Part print with two shaded views. Sizes in mm from the minimum x, y, z corner. A direction names the side the tool comes from. Round coordinates to 2 decimals unless told otherwise and drop trailing zeros. Write each loop counter-clockwise with the first axis right and the second up, starting at its lowest first coordinate (ties: lowest second). Pieces come first, ordered by that corner, then holes. Notation, with made-up numbers: (-14, 53.5) - (0, 53.5) arc R17 ccw to (0, 71.5) - close; hole circle Ø6 at (73, 79.5). An arc over 180 degrees is marked (long way). Answer as a JSON object with one key per item and string values. Group by question number.
Item 1: Slice it at B-B, the plane x = 522.5. List the corners of the cut face in (y, z).
Item 2: Two-plate mould, pull along Y, no slides. Class the marked faces 3, 4, 5 and 6: +Y half, -Y half, draft (parallel to the pull), parting line (faces both ways), or undercut.
Item 3: Flat gauge pin, fed straight in: pin 1 (10 mm diameter, centred on x = 379.5, y = 118, fed in from +Z). Where does the tip first touch, or does it go through?
Item 4: Slice it at D-D, the plane x = 293.5. List the corners of the cut face in (y, z).
Item 5: Slice it at A-A, the plane y = 49. List the corners of the cut face in (x, z), then the cut area to 3 significant figures.
Item 6: Slice it at C-C, the plane z = 130.5. List the corners of the cut face in (x, y), then the cut area to 3 significant figures.
Item 7: Probe line 1 (Y direction, x = 104, z = 51); line 2 (X direction, y = 137.5, z = 66); line 3 (Z direction, x = 210.5, y = 37.5). List the from-to ranges inside material, lowest first. Write a range as from..to.
Item 8: Which spindle directions (+Z, -Z, +X, -X, +Y, -Y) get a long thin tool onto all of the face, cutting with end or side? Do the marked faces 1 and 2. Say none if no direction does.
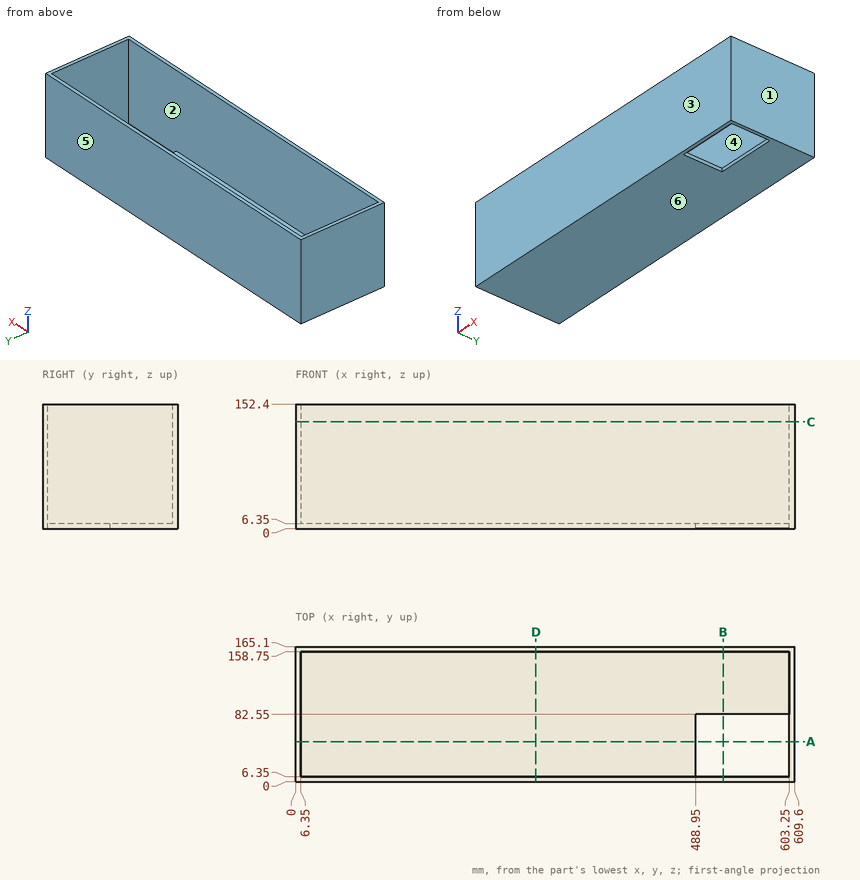
Geometry says:
{
 "1": {"outline": "(0, 0) - (6.35, 0) - (6.35, 152.4) - (0, 152.4) - close; (82.55, 0) - (165.1, 0) - (165.1, 152.4) - (158.75, 152.4) - (158.75, 6.35) - (82.55, 6.35) - close"},
 "2": {"face 3": "-Y half", "face 4": "undercut", "face 5": "+Y half", "face 6": "draft"},
 "3": {"pin 1": "stops at z = 6.35"},
 "4": {"outline": "(0, 0) - (165.1, 0) - (165.1, 152.4) - (158.75, 152.4) - (158.75, 6.35) - (6.35, 6.35) - (6.35, 152.4) - (0, 152.4) - close"},
 "5": {"outline": "(0, 0) - (488.95, 0) - (488.95, 6.35) - (6.35, 6.35) - (6.35, 152.4) - (0, 152.4) - close; (603.25, 0) - (609.6, 0) - (609.6, 152.4) - (603.25, 152.4) - close", "area": "5,000 mm^2"},
 "6": {"outline": "(0, 0) - (609.6, 0) - (609.6, 165.1) - (0, 165.1) - close; hole (6.35, 6.35) - (603.25, 6.35) - (603.25, 158.75) - (6.35, 158.75) - close", "area": "9,680 mm^2"},
 "7": {"line 1": "y = 0..6.35, 158.75..165.1", "line 2": "x = 0..6.35, 603.25..609.6", "line 3": "z = 0..6.35"},
 "8": {"face 1": "+Z, -Z, +X, +Y, -Y", "face 2": "+Z"}
}
